The listing builds one solid part. Answer for the finished solid, in the listing's coordinates (mm). A direction names the side the tool comes from. Round coordinates to 2 decimals unless told otherwise and drop trailing zeros. Write each loop counter-clockwise with the first axis right and the second up, starting at its lowest first coordinate (ties: lowest second). Pieces come first, ordered by that corner, then holes. Notation, with made-up numbers: (22.5, 31) - (52.5, 31) arc R29 cw to (52.5, 69) - close; hole circle Ø10 at (-38.75, 22.25). An arc over 180 degrees is marked (long way). Use a Markdown table: item, result. Add a question column.
1) Find the intervals of material crossed by probe 1 along X at (y, z) = (36.83, 1.05); probe 2 along X at (y, z) = (96.52, 1.25); probe 3 along Y at (x, z) = (45.72, 0.4), in increasing order. Write a range as from..to.
2) A cutting plane is placed at A-A (x = 45.72). Give the vertices of the cut face in (y, z), then the cut area to 3 significant figures.
3) Each of these flat-tipped pins is pushed along its axis until it touches: P1, Ø3.5, axis at x = 110.744, y = 37.084, coming from the +Z side; P2, Ø0.5, axis at x = 53.5, z = 0.5, coming from the +Y side; P3, Ø0.5, axis at y = 88, z = 1, coming from the -X side. Where does it stop, or does it pass through?
4) A cutting plane is placed at B-B (y = 36.83). Give the vertices of the cut face in (x, z), then the cut area to 3 significant figures.
5) A cutting plane is placed at D-D (x = 59). Give the vertices of the cut face in (y, z), then the cut area to 3 significant figures.
6) Determine the mould class of faces 3 (the flat face through (58, 85.09, 1)), 4 (the cylindrical face through (109.645, 38.282, 0.798)), 5 (the flat face through (78, 69, 0)) for opening direction Y: +Y half, -Y half, draft (parallel to the pull), parting line (faces both ways), or undercut.
7) A cutting plane is placed at C-C (z = 0.9). State how many separate pieces and enclosed holes the cut face has, then the cut area to 3 significant figures.
8) A tool of negligible diameter and unlimited length cuts with its end or side. For faces 1 (the flat face through (73.66, 89, 1)), 2 (the flat face through (79, 34.29, 1)), from which of +Z, -Z, +X, -X, +Y, -Y can it reach the whole face along a straight path? Write none if from no direction.
Autodesk Inventor part; units mm, degrees
ref_plane "BoardFrontPlane" through (0, 0, 0) normal (0, 0, 1) x (1, 0, 0)
ref_plane "YZ Plane" through (0, 0, 0) normal (1, 0, 0) x (0, 1, 0)
ref_plane "XZ Plane" through (0, 0, 0) normal (0, 1, 0) x (-1, 0, 0)
ref_plane "BoardFrontPlane" through (0, 0, 0) normal (0, 0, 1) x (1, 0, 0)
sketch "Sketch1" plane through (0, 0, 0) normal (0, 0, 1) x (1, 0, 0)
  line L0 (43.18, 34.29) -> (43.18, 85.09)
  line L1 (43.18, 85.09) -> (73.66, 85.09)
  line L2 (73.66, 85.09) -> (73.66, 93.98)
  line L3 (73.66, 93.98) -> (82.55, 102.87)
  line L4 (82.55, 102.87) -> (113.284, 102.87)
  line L5 (113.284, 102.87) -> (113.284, 34.29)
  line L6 (113.284, 34.29) -> (43.18, 34.29)
extrude "BoardOutline" add sketch "Sketch1" along normal blind 1.6194
sketch "img_Top" plane through (0, 0, 1.6194) normal (0, 0, 1) x (1, 0, 0)
  line L0 (43.18, 102.87) -> (113.284, 102.87) construction
  line L1 (113.284, 102.87) -> (113.284, 34.29) construction
  line L2 (113.284, 34.29) -> (43.18, 34.29) construction
  line L3 (43.18, 34.29) -> (43.18, 102.87) construction
decal "Decal_Top"
sketch "img_Bottom" plane through (0, 0, -1.6194) normal (0, 0, -1) x (1, 0, 0)
  line L0 (43.18, -34.29) -> (113.284, -34.29) construction
  line L1 (113.284, -34.29) -> (113.284, -102.87) construction
  line L2 (113.284, -102.87) -> (43.18, -102.87) construction
  line L3 (43.18, -102.87) -> (43.18, -34.29) construction
decal "Decal_Bottom"
sketch "Sketch4" plane through (0, 0, 1.6194) normal (0, 0, 1) x (1, 0, 0)
  point P0 (94.234, 97.79)
hole "SW301-H1" at (94.234, 97.79, 1.6194) direction (0, 0, -1) diameter 0.85 end through all
sketch "Sketch5" plane through (0, 0, 1.6194) normal (0, 0, 1) x (1, 0, 0)
  point P0 (106.934, 95.25)
hole "SW300-H1" at (106.934, 95.25, 1.6194) direction (0, 0, -1) diameter 0.85 end through all
sketch "Sketch6" plane through (0, 0, 1.6194) normal (0, 0, 1) x (1, 0, 0)
  point P0 (45.72, 36.83)
hole "Free-MNT+4" at (45.72, 36.83, 1.6194) direction (0, 0, -1) diameter 3.2512 end through all
sketch "Sketch7" plane through (0, 0, 1.6194) normal (0, 0, 1) x (1, 0, 0)
  point P0 (110.744, 37.084)
hole "Free-MNT+3" at (110.744, 37.084, 1.6194) direction (0, 0, -1) diameter 3.2512 end through all
sketch "Sketch8" plane through (0, 0, 1.6194) normal (0, 0, 1) x (1, 0, 0)
  point P0 (110.744, 100.076)
hole "Free-MNT+2" at (110.744, 100.076, 1.6194) direction (0, 0, -1) diameter 3.2512 end through all
sketch "Sketch9" plane through (0, 0, 1.6194) normal (0, 0, 1) x (1, 0, 0)
  point P0 (90.805, 96.52)
hole "JP300-1" at (90.805, 96.52, 1.6194) direction (0, 0, -1) diameter 1.016 end through all
sketch "Sketch10" plane through (0, 0, 1.6194) normal (0, 0, 1) x (1, 0, 0)
  point P0 (88.265, 96.52)
hole "JP300-2" at (88.265, 96.52, 1.6194) direction (0, 0, -1) diameter 1.016 end through all
sketch "Sketch11" plane through (0, 0, 1.6194) normal (0, 0, 1) x (1, 0, 0)
  point P0 (85.725, 96.52)
hole "JP300-3" at (85.725, 96.52, 1.6194) direction (0, 0, -1) diameter 1.016 end through all
sketch "Sketch12" plane through (0, 0, 1.6194) normal (0, 0, 1) x (1, 0, 0)
  point P0 (83.185, 96.52)
hole "JP300-4" at (83.185, 96.52, 1.6194) direction (0, 0, -1) diameter 1.016 end through all
sketch "Sketch13" plane through (0, 0, 1.6194) normal (0, 0, 1) x (1, 0, 0)
  point P0 (94.996, 91.44)
hole "J300-_OMJMIDLA" at (94.996, 91.44, 1.6194) direction (0, 0, -1) diameter 0.9 end through all
sketch "Sketch14" plane through (0, 0, 1.6194) normal (0, 0, 1) x (1, 0, 0)
  point P0 (94.996, 89.408)
hole "J300-_YAKUTFXJ" at (94.996, 89.408, 1.6194) direction (0, 0, -1) diameter 0.9 end through all
sketch "Sketch15" plane through (0, 0, 1.6194) normal (0, 0, 1) x (1, 0, 0)
  point P0 (100.076, 90.424)
hole "J300-_MBXSYRVB" at (100.076, 90.424, 1.6194) direction (0, 0, -1) diameter 0.9 end through all
properties part number "skimmer_swabbie_v1_BOARD"
Entries:
| question | item | result |
|---|---|---|
| 1 | probe 1 | x = 43.18..44.09, 47.35..109.14, 112.35..113.28 |
| 1 | probe 2 | x = 76.2..82.68, 83.69..85.22, 86.23..87.76, 88.77..90.3, 91.31..113.28 |
| 1 | probe 3 | y = 34.29..35.2, 38.46..85.09 |
| 2 | outline | (34.29, 0) - (35.2, 0) - (35.2, 1.62) - (34.29, 1.62) - close; (38.46, 0) - (85.09, 0) - (85.09, 1.62) - (38.46, 1.62) - close |
| 2 | area | 77.0 mm² |
| 3 | P1 | stops at z = 1.62 |
| 3 | P2 | stops at y = 85.09 |
| 3 | P3 | stops at x = 73.66 |
| 4 | outline | (43.18, 0) - (44.09, 0) - (44.09, 1.62) - (43.18, 1.62) - close; (47.35, 0) - (109.14, 0) - (109.14, 1.62) - (47.35, 1.62) - close; (112.35, 0) - (113.28, 0) - (113.28, 1.62) - (112.35, 1.62) - close |
| 4 | area | 103 mm² |
| 5 | outline | (34.29, 0) - (85.09, 0) - (85.09, 1.62) - (34.29, 1.62) - close |
| 5 | area | 82.3 mm² |
| 6 | face 3 | +Y half |
| 6 | face 4 | undercut |
| 6 | face 5 | draft |
| 7 | separate pieces | 1 |
| 7 | enclosed holes | 12 |
| 7 | area | 4,200 mm² |
| 8 | face 1 | +Z, -Z, -X, +Y |
| 8 | face 2 | +Z, -Z, +X, -X, -Y |
